from build123d import *

# Parameters (mm, degrees)
F0_W     = 6
F0_H     = 7.6
F0_R     = 1.6
F0_W_2   = 0.25
F0_W_3   = 21
F1_DEPTH = 4
F2_DEPTH = 1.2
F3_R     = 1


with BuildPart() as f1:
    # F0 (on Top) → F1 (new body)
    with BuildSketch(Plane.XY):
        with Locations((-13.75, 0)):
            Rectangle(F0_W, F0_H)
        with Locations((-13.75, 0)):
            Circle(F0_R, mode=Mode.SUBTRACT)
        with Locations((13.75, 0)):
            Rectangle(F0_W, F0_H)
        with Locations((13.75, 0)):
            Circle(F0_R, mode=Mode.SUBTRACT)
        with Locations((-10.625, 0)):
            Rectangle(F0_W_2, F0_H)
        Rectangle(F0_W_3, F0_H)
        with Locations((10.625, 0)):
            Rectangle(F0_W_2, F0_H)
    extrude(amount=F1_DEPTH)

    # F0 (on Top) → F2 (cut)
    with BuildSketch(Plane.XY):
        Rectangle(F0_W_3, F0_H)
    extrude(amount=F2_DEPTH, mode=Mode.SUBTRACT)

    # F3
    f3_edges = [f1.edges().sort_by_distance(p)[0] for p in [
        (-13.625, -3.8, 0),
        (-10.5, -3.8, 0.6),
        (0, -3.8, 1.2),
        (10.5, -3.8, 0.6),
        (13.625, -3.8, 0),
        (16.75, -3.8, 2),
        (0, -3.8, 4),
        (-16.75, -3.8, 2),
        (-16.75, 3.8, 2),
        (0, 3.8, 4),
        (16.75, 3.8, 2),
        (13.625, 3.8, 0),
        (10.5, 3.8, 0.6),
        (0, 3.8, 1.2),
        (-10.5, 3.8, 0.6),
        (-13.625, 3.8, 0),
        (16.75, 0, 0),
        (16.75, 0, 4),
        (-16.75, 0, 0),
        (-16.75, 0, 4),
    ]]
    fillet(f3_edges, radius=F3_R)


solid = f1.part
Geometry: final body of the model. Coordinates: model frame, mm. A direction names the side the tool comes from. Give positions to 0.01 mm unless a question says otherwise; leave off trailing zeros. Loops run counter-clockwise (first coordinate to the right, second up) from the corner with the lowest first, then second, coordinate; pieces in that order, holes last. Notation, with made-up numbers: (-27.5, 48) - (0.5, 48) arc R28 ccw to (0.5, 83) - close; hole circle Ø8 at (31, 34.5). An arc over 180 degrees is marked (long way). One line per question, with ' | ' between items. Start each with the question number.
(1) Section query B-B on z = 0.4. Return loops of the section in (x, y), then the cut area to 3 significant figures.
(2) Section query D-D on z = 2.65. Return loops of the section in (x, y).
(3) Section query C-C on y = 0. Return loops of the section in (x, z).
(4) Reachability of faces 4 (the flat face through (-10.5, 0, 1)), 5 (the cylindrical face through (10.801, -3.515, 0.871)), 6 (the cylindrical face through (0.161, 3.515, 1.501)) from +Z, -Z, +X, -X, +Y, -Y: full face, straight path, thin tool, end or side. Return the list, or none.
(5) Section query A-A on x = -13.75. Return loops of the section in (y, z).
(6) Pull-direction query (X, two-part tool) for faces 1 (the flat face through (-16.75, 0, 2)), 2 (the cylindrical face through (-13.162, 3.515, 0.301)), 3 (the cylindrical face through (-15.35, 0.07, 1.97)); classes: released by +X, released by -X, zero draft, split by the parting line, or undercut.
(7) Ray query, line 1 (Y direction, x = 13.75, z = 3); line 2 (X direction, y = -1, z = 0.2); line 3 (Y direction, x = -4.5, z = 3.05). Return the intervals inside material, ascending. Write a range as from..to.
(8) Contact query for a flat-ended pin moving along its axis: pin 1 (2 mm diameter, centred on x = 5, y = 0, fed in from -Z). Output: stop coordinate, or through.
The answers:
1) outline: (-16.55, -2.8) arc R0.8 ccw to (-15.75, -3.6) - (-10.9, -3.6) arc R1 ccw to (-10.5, -2.8) - (-10.5, 2.8) arc R1 ccw to (-10.9, 3.6) - (-15.75, 3.6) arc R0.8 ccw to (-16.55, 2.8) - close; (10.5, -2.8) arc R1 ccw to (10.9, -3.6) - (15.75, -3.6) arc R0.8 ccw to (16.55, -2.8) - (16.55, 2.8) arc R0.8 ccw to (15.75, 3.6) - (10.9, 3.6) arc R1 ccw to (10.5, 2.8) - close; hole circle Ø3.2 at (-13.75, 0); hole circle Ø3.2 at (13.75, 0) | area: 70.1 mm2
2) outline: (-16.75, -2.8) arc R1 ccw to (-15.75, -3.8) - (15.75, -3.8) arc R1 ccw to (16.75, -2.8) - (16.75, 2.8) arc R1 ccw to (15.75, 3.8) - (-15.75, 3.8) arc R1 ccw to (-16.75, 2.8) - close; hole circle Ø3.2 at (-13.75, 0); hole circle Ø3.2 at (13.75, 0)
3) outline: (-16.75, 1) arc R1 ccw to (-15.75, 0) - (-15.35, 0) - (-15.35, 4) - (-15.75, 4) arc R1 ccw to (-16.75, 3) - close; (-12.15, 0) - (-10.5, 0) - (-10.5, 1.2) - (10.5, 1.2) - (10.5, 0) - (12.15, 0) - (12.15, 4) - (-12.15, 4) - close; (15.35, 0) - (15.75, 0) arc R1 ccw to (16.75, 1) - (16.75, 3) arc R1 ccw to (15.75, 4) - (15.35, 4) - close
4) face 4: -Z, +Y, -Y | face 5: -Z, -Y | face 6: -Z, +Y
5) outline: (-3.8, 1) arc R1 ccw to (-2.8, 0) - (-1.6, 0) - (-1.6, 4) - (-2.8, 4) arc R1 ccw to (-3.8, 3) - close; (1.6, 0) - (2.8, 0) arc R1 ccw to (3.8, 1) - (3.8, 3) arc R1 ccw to (2.8, 4) - (1.6, 4) - close
6) face 1: released by -X | face 2: zero draft | face 3: undercut
7) line 1: -3.8..-1.6, 1.6..3.8 | line 2: -16.35..-15, -12.5..-10.5, 10.5..12.5, 15..16.35 | line 3: -3.8..3.8
8) pin 1: z = 1.2
